The listing builds one solid part. Answer for the finished solid, in the listing's coordinates (mm). Round coordinates to 2 decimals unless told otherwise and drop trailing zeros. Write each loop counter-clockwise with the first axis right and the second up, starting at its lowest first coordinate (ties: lowest second). Pieces come first, ordered by that corner, then holes. Notation, with made-up numbers: (81.5, 76) - (116.5, 76) arc R15 cw to (116.5, 99) - close; hole circle Ø10 at (-19.75, -1.5). An arc over 180 degrees is marked (long way). Use a Markdown table: item, result. Add a question column.
1) A cutting plane is placed at B-B (x = 3.5). Give the vertices of the cut face in (y, z) (3 decimals).
2) A cutting plane is placed at A-A (x = 39). Give the vertices of the cut face in (y, z).
3) Determine the mould class of faces 1 (the flat face through (54, 1.753, -46)), 2 (the cylindrical face through (38.72, 0.89, -53.76)) for opening direction X: +X half, -X half, draft (parallel to the pull), parting line (faces both ways), or undercut.
4) Find the intervals of material crossed by probe 1 along Z at (x, y) = (53.5, 0.4) (3 decimals); probe 2 along X at (y, z) = (1.2, -9.8); probe 3 along Z at (x, y) = (3.5, 0.4) (3 decimals), in increasing order. Write a range as from..to.
5) A cutting plane is placed at C-C (y = 1.4). State how many separate pieces and enclosed holes the cut face has, then the cut area to 3 significant figures.
6) Each of these flat-tipped pins is pushed along its axis until it touches: P1, Ø3.5, axis at x = 3.5, z = -45, coming from the +Y side; P2, Ø0.9, axis at x = 107.5, y = 1, coming from the -Z side. Where does it stop, or does it pass through?
```python
from build123d import *

# Parameters (mm, degrees)
FR4_DEPTH                           = 1.7526
SKETCH7_R                           = 1.905
THERMAL_WALL_HOLES_SIDES_DEPTH      = 2.7526
SKETCH8_R                           = 0.47
SKETCH8_R_2                         = 0.33
CONTROLLED_DEPTH_HOLES_TOP_DEPTH    = 1.1176
SKETCH9_R                           = 0.47
SKETCH9_R_2                         = 0.32
SKETCH9_R_3                         = 0.33
CONTROLLED_DEPTH_HOLES_BOTTOM_DEPTH = 1.1176
SKETCH10_R                          = 1.27
THERMAL_SCREW_HOLES_MIDDLE_DEPTH    = 2.7526


with BuildPart() as part:
    # Sketch1 → FR4 (new body)
    with BuildSketch(Plane(origin=(0, 0, 0), x_dir=(1, 0, 0), z_dir=(0, 1, 0))):
        with BuildLine():
            Line((0, 0), (110, 0))
            Line((110, 0), (110, 87))
            Line((110, 87), (104, 87))
            ThreePointArc((104, 87), (102.585786438, 87.585786438), (102, 89))
            Line((102, 89), (102, 89.75))
            Line((102, 89.75), (64, 89.75))
            Line((64, 89.75), (64, 88.5))
            ThreePointArc((64, 88.5), (63.414213562, 87.085786438), (62, 86.5))
            Line((62, 86.5), (48, 86.5))
            ThreePointArc((48, 86.5), (46.585786438, 87.085786438), (46, 88.5))
            Line((46, 88.5), (46, 89.75))
            Line((46, 89.75), (8, 89.75))
            Line((8, 89.75), (8, 89))
            ThreePointArc((8, 89), (7.414213562, 87.585786438), (6, 87))
            Line((6, 87), (0, 87))
            Line((0, 87), (0, 0))
        make_face()
    extrude(amount=FR4_DEPTH)

    # Sketch7 → thermal-wall-holes-sides (cut, through all)
    with BuildSketch(Plane(origin=(0, 1.7526, 0), x_dir=(1, 0, 0), z_dir=(0, 1, 0))):
        with Locations((3.5, 15)):
            Circle(SKETCH7_R)
        with Locations((106.5, 15)):
            Circle(SKETCH7_R)
        with Locations((106.5, 30)):
            Circle(SKETCH7_R)
        with Locations((106.5, 45)):
            Circle(SKETCH7_R)
        with Locations((106.5, 60)):
            Circle(SKETCH7_R)
        with Locations((106.5, 75)):
            Circle(SKETCH7_R)
        with Locations((3.5, 30)):
            Circle(SKETCH7_R)
        with Locations((3.5, 45)):
            Circle(SKETCH7_R)
        with Locations((3.5, 60)):
            Circle(SKETCH7_R)
        with Locations((3.5, 75)):
            Circle(SKETCH7_R)
    extrude(amount=-THERMAL_WALL_HOLES_SIDES_DEPTH, mode=Mode.SUBTRACT)

    # Sketch8 → controlled-depth-holes.top (cut)
    with BuildSketch(Plane(origin=(0, 1.7526, 0), x_dir=(1, 0, 0), z_dir=(0, 1, 0))):
        with Locations((8.9, 9.8)):
            Circle(SKETCH8_R)
        with Locations((66.9, 9.8)):
            Circle(SKETCH8_R)
        with Locations((53.2, 50.9)):
            Circle(SKETCH8_R)
        with Locations((53.2, 85.1)):
            Circle(SKETCH8_R_2)
        with Locations((43.1, 9.8)):
            Circle(SKETCH8_R_2)
        with Locations((101.1, 9.8)):
            Circle(SKETCH8_R_2)
    extrude(amount=-CONTROLLED_DEPTH_HOLES_TOP_DEPTH, mode=Mode.SUBTRACT)

    # Sketch9 → controlled-depth-holes.bottom (cut)
    with BuildSketch(Plane.XZ):
        with Locations((8.975, -9.5)):
            Circle(SKETCH9_R)
        with Locations((66.975, -9.5)):
            Circle(SKETCH9_R)
        with Locations((53.5, -50.975)):
            Circle(SKETCH9_R)
        with Locations((53.5, -85.175)):
            Circle(SKETCH9_R_2)
        with Locations((43.175, -9.5)):
            Circle(SKETCH9_R_3)
        with Locations((101.175, -9.5)):
            Circle(SKETCH9_R_3)
    extrude(amount=-CONTROLLED_DEPTH_HOLES_BOTTOM_DEPTH, mode=Mode.SUBTRACT)

    # Sketch10 → thermal-screw-holes-middle (cut, through all)
    with BuildSketch(Plane(origin=(0, 1.7526, 0), x_dir=(1, 0, 0), z_dir=(0, 1, 0))):
        with Locations((39, 55)):
            Circle(SKETCH10_R)
        with Locations((71, 55)):
            Circle(SKETCH10_R)
        with Locations((71, 35)):
            Circle(SKETCH10_R)
        with Locations((39, 35)):
            Circle(SKETCH10_R)
    extrude(amount=-THERMAL_SCREW_HOLES_MIDDLE_DEPTH, mode=Mode.SUBTRACT)


solid = part.part
```
Entries:
| question | item | result |
|---|---|---|
| 1 | outline | (0, -87) - (1.753, -87) - (1.753, -76.905) - (0, -76.905) - close; (0, -73.095) - (1.753, -73.095) - (1.753, -61.905) - (0, -61.905) - close; (0, -58.095) - (1.753, -58.095) - (1.753, -46.905) - (0, -46.905) - close; (0, -43.095) - (1.753, -43.095) - (1.753, -31.905) - (0, -31.905) - close; (0, -28.095) - (1.753, -28.095) - (1.753, -16.905) - (0, -16.905) - close; (0, -13.095) - (1.753, -13.095) - (1.753, 0) - (0, 0) - close |
| 2 | outline | (0, -89.75) - (1.75, -89.75) - (1.75, -56.27) - (0, -56.27) - close; (0, -53.73) - (1.75, -53.73) - (1.75, -36.27) - (0, -36.27) - close; (0, -33.73) - (1.75, -33.73) - (1.75, 0) - (0, 0) - close |
| 3 | face 1 | draft |
| 3 | face 2 | undercut |
| 4 | probe 1 | z = -86.5..-85.495, -84.855..-51.445, -50.505..0 |
| 4 | probe 2 | x = 0..8.43, 9.37..42.77, 43.43..66.43, 67.37..100.77, 101.43..110 |
| 4 | probe 3 | z = -87..-76.905, -73.095..-61.905, -58.095..-46.905, -43.095..-31.905, -28.095..-16.905, -13.095..0 |
| 5 | separate pieces | 1 |
| 5 | enclosed holes | 20 |
| 5 | area | 9,640 mm² |
| 6 | P1 | passes through |
| 6 | P2 | stops at z = -87 |
